Can you work these out from the model? Positions are in its coordinate system, mm. Round coordinates to 2 decimals unless told otherwise and drop trailing zeros. Write each loop counter-clockwise with the first axis right and the second up, starting at its lowest first coordinate (ties: lowest second). Pieces come first, ordered by that corner, then holes. Notation, with made-up numbers: M 2,-6 L 31,-6 A22 ccw 31,30 Z; hole C 86,81.25 d10. An arc over 180 degrees is marked long. Answer in a Markdown table with one row per item. Add a question column.
(1) Suppose I cut it at A-A, the plane y = 0. Write out the boundary of the cut face in (x, z), then the cut area to 3 significant figures.
(2) If we mould it in two halves opening along X, with no side actions, what happens to faces 1 (the face through (-50, 26, 0)), 2 (the face through (55.534, 66.198, 6.084)), 3 (the face through (-23.846, 107.384, 5.916))? For each: released by +X, released by -X, zero draft, split by the parting line, or undercut.
(3) Suppose I cut it at C-C, the plane y = -36.5. Write out the boundary of the cut face in (x, z).
(4) If I drill on probe 1 along X at (y, z) = (65, 3.75); probe 2 along X at (y, z) = (63, 9.5); probe 3 along Y at (x, z) = (71, 3.75), over which ranges is the centre line in solid material (lowest first)?
(5) Suppose I cut it at D-D, the plane x = -66. Write out the boundary of the cut face in (y, z), then the cut area to 3 significant figures.
(6) Suppose I cut it at B-B, the plane x = -23.5. Write out the boundary of the cut face in (y, z), then the cut area to 3 significant figures.
(7) I'm going to push flat-ended pins straight in: pin 1 (5 mm diameter, centred on x = -69, z = 2, fed in from -Y); pin 2 (5 mm diameter, centred on y = -16.5, z = 1.5, fed in from -X); pin 3 (1 mm diameter, centred on y = -39, z = 7, fed in from -X); pin 4 (22 mm diameter, centred on x = -63.64, y = -63.64, fed in from +Z). Where does each tip first touch, or does it pass through?
Autodesk Inventor part; units mm, degrees
ref_plane "YZ Plane" through (0, 0, 0) normal (1, 0, 0) x (0, 1, 0)
ref_plane "XZ Plane" through (0, 0, 0) normal (0, 1, 0) x (-1, 0, 0)
ref_plane "XY Plane" through (0, 0, 0) normal (0, 0, 1) x (1, 0, 0)
sketch "Sketch2" plane through (0, 0, 0) normal (0, 0, 1) x (1, 0, 0)
  circle A0 centre (0, 0) radius 56
  circle A1 centre (0, 0) radius 110
  dimension "d25" = 112
  dimension "d27" = 220
extrude "Plate2" add sketch "Sketch2" along normal blind 12
sketch "Sketch3" plane through (0, 0, 12) normal (0, 0, 1) x (1, 0, 0)
  circle A0 centre (-90, 0) radius 8.5
  circle A1 centre (0, 0) radius 90 construction
  dimension "d28" = 180
  dimension "d15" = 17
extrude "Cut1" cut sketch "Sketch3" against normal blind 12
pattern_circular "Circular Pattern1" count 8 over 360 about axis through (0, 0, -10) along (0, 0, 1) of "Cut1"
equation "\"d17\" = Thickness"
equation "\"d14\" = Thickness"
equation "\"BendReliefWidth\" = Thickness"
equation "\"BendReliefDepth\" = 0.5 * Thickness"
equation "\"CornerReliefSize\" = 4 * Thickness"
equation "\"MinimumRemnant\" = 2 * Thickness"
equation "\"TransitionRadius\" = BendRadius"
equation "\"JacobiRadiusSize\" = BendRadius"
equation "\"GapSize\" = Thickness"
properties part number "APN 1433 FDS flange DN100" material "Steel"
Calculated:
| question | item | result |
|---|---|---|
| 1 | outline | M -110,0 L -98.5,0 L -98.5,12 L -110,12 Z; M -81.5,0 L -56,0 L -56,12 L -81.5,12 Z; M 56,0 L 81.5,0 L 81.5,12 L 56,12 Z; M 98.5,0 L 110,0 L 110,12 L 98.5,12 Z |
| 1 | area | 888 mm² |
| 2 | face 1 | zero draft |
| 2 | face 2 | undercut |
| 2 | face 3 | split by the parting line |
| 3 | outline | M -103.77,0 L -42.47,0 L -42.47,12 L -103.77,12 Z; M 42.47,0 L 103.77,0 L 103.77,12 L 42.47,12 Z |
| 4 | probe 1 | -88.74 to -72.03, -55.25 to 55.25, 72.03 to 88.74 |
| 4 | probe 2 | -90.17 to -72.12, -55.16 to 55.16, 72.12 to 90.17 |
| 4 | probe 3 | -84.02 to -67.89, -59.39 to 59.39, 67.89 to 84.02 |
| 5 | outline | M -88,0 L -71.81,0 L -71.81,12 L -88,12 Z; M -55.47,0 L 55.47,0 L 55.47,12 L -55.47,12 Z; M 71.81,0 L 88,0 L 88,12 L 71.81,12 Z |
| 5 | area | 1,720 mm² |
| 6 | outline | M -107.46,0 L -50.83,0 L -50.83,12 L -107.46,12 Z; M 50.83,0 L 107.46,0 L 107.46,12 L 50.83,12 Z |
| 6 | area | 1,360 mm² |
| 7 | pin 1 | y = -87.62 |
| 7 | pin 2 | x = -109.11 |
| 7 | pin 3 | x = -103.04 |
| 7 | pin 4 | z = 12 |
